Could you check a few things on this model? Use its own coordinates, in mm. A direction names the side the tool comes from. Give positions to 0.01 mm unless a question says otherwise; leave off trailing zeros. Order: outer loops, then holes, each group sorted by start corner. A loop starts at its lowest first (then second) coordinate and runs counter-clockwise, first axis right, second up. Notation, with made-up numbers: (-33.75, 58) -> (-26.75, 58) arc R10 ccw to (-26.75, 70) -> close; hole circle Ø10 at (85, 38). An arc over 180 degrees is marked (long way). Answer as CSV lines item,"result". Start each with the question number.
(1) I want a section at A-A (z = 158). Please give me the cut outline in (x, y).
(2) Will these pins go through, and if not, where does the flat tip stop? pin 1 Ø4 at (x, z) = (3.5, 121) entering from +Y; pin 2 Ø2 at (x, z) = (2.5, 282) entering from -Y.
(3) I need wall thicknesses on L1, parallel to Y at x = -0.25, z = 362; L2, parallel to X at y = 4.5, z = 294.5. Which ranges of each line are inside material? Lowest first, please.
(4) On a 3-axis mill with a long thin cutter (end or side, diameter ignored), from which of +Z, -Z, +X, -X, +Y, -Y can I reach the whole of each face in a straight line? I mean faces 1 (the face through (0.867, 3.905, 5.563)), 2 (the face through (-6, 0, 193)). Say none if no direction works.
```python
from build123d import *

# Parameters (mm, degrees)
SCHIZZO1_R                   = 6
ESTRUSIONE_ESTRUSIONE1_DEPTH = 380
SMUSSO1_SIZE                 = 1


with BuildPart() as part:
    # Schizzo1 → Estrusione-Estrusione1 (new body)
    with BuildSketch(Plane.XY):
        Circle(SCHIZZO1_R)
    extrude(amount=ESTRUSIONE_ESTRUSIONE1_DEPTH)

    # Schizzo2 → Taglia-Rivoluzione1 (revolve, cut)
    with BuildSketch(Plane(origin=(0, 0, 0), x_dir=(1, 0, 0), z_dir=(0, 1, 0))):
        Polygon((-4, -10), (-6, -12), (-6, 0), (-4, 0), align=None)
    revolve(axis=Axis((0, 0, -1.898721367), (0, 0, 1)), mode=Mode.SUBTRACT)

    # Smusso1
    smusso1_edges = [part.edges().sort_by_distance(p)[0] for p in [
        (-6, 0, 380),
        (4, 0, 0),
    ]]
    chamfer(smusso1_edges, length=SMUSSO1_SIZE)


solid = part.part
```
Final values:
1,outline,"circle Ø12 at (0, 0)"
2,pin 1,"y = 5.81"
2,pin 2,"y = -5.81"
3,L1,"-5.99 to 5.99"
3,L2,"-3.97 to 3.97"
4,face 1,"-Z"
4,face 2,"+Z, -Z"
